Verification items for the finished model (mm, model axes). Coordinates: 2 decimals unless noted, no trailing zeros. Write each loop counter-clockwise with the first axis right and the second up, starting at its lowest first coordinate (ties: lowest second). Pieces come first, ordered by that corner, then holes. Notation, with made-up numbers: (-12.75, -21.75) -> (9.25, -21.75) arc R20 ccw to (9.25, 4.25) -> close; hole circle Ø6 at (79, 23). An arc over 180 degrees is marked (long way). Use CSV: the item, a comma, the result in double quotes.
Autodesk Inventor part; units mm, degrees
ref_plane "YZ Plane" through (0, 0, 0) normal (1, 0, 0) x (0, 1, 0)
ref_plane "XZ Plane" through (0, 0, 0) normal (0, 1, 0) x (-1, 0, 0)
ref_plane "XY Plane" through (0, 0, 0) normal (0, 0, 1) x (1, 0, 0)
sketch "Sketch1" plane through (0, 0, 0) normal (0, 0, 1) x (1, 0, 0)
  line L0 (51.9615, 90) -> (103.923, 0)
  line L1 (103.923, 0) -> (51.9615, -90)
  line L2 (51.9615, -90) -> (-51.9615, -90)
  line L3 (-51.9615, -90) -> (-103.923, 0)
  line L4 (-103.923, 0) -> (-51.9615, 90)
  line L5 (-51.9615, 90) -> (51.9615, 90)
  circle A0 centre (0, 0) radius 85
  circle A1 centre (0, 0) radius 10
  dimension "d1" = 170
  dimension "d2" = 180
  dimension "d12" = 20
extrude "Extrusion1" add sketch "Sketch1" along normal blind 1.6 contours L0 L1 L2 L3 L4 L5 | A0
sketch "Sketch3" plane through (0, 0, 1.6) normal (0, 0, 1) x (1, 0, 0)
  circle A0 centre (0, 0) radius 10
  circle A1 centre (-96, 0) radius 1.6
  line L0 (-51.9615, 90) -> (-103.923, 0)
  line L1 (-103.923, 0) -> (-51.9615, -90)
  arc A2 (-101.2676, 4.5994) -> (-101.2676, -4.5994) centre (-93.3013, 0) ccw
  dimension "d13" = 96
  dimension "d14" = 3.2
  dimension "d20" = 9.1987
  dimension "d21" = 93.3013
extrude "Extrusion3" cut sketch "Sketch3" against normal up to next contours A1 | A2 L1 L0
pattern_circular "Circular Pattern1" count 6 over 360 about axis through (0, 0, 0) along (0, 0, 1) of "Extrusion3"
sketch "Sketch4" plane through (0, 0, 1.6) normal (0, 0, 1) x (1, 0, 0)
  circle A0 centre (0, 0) radius 10
  circle A1 centre (0, 0) radius 85
  dimension "d22" = 170
extrude "Extrusion4" add sketch "Sketch4" along normal blind 0.1
properties part number "Heatbed_170mm_Hex"
1) Cross-section at C-C (x = -88). Record the boundary of the cut face in (y, z), plus the area to 3 significant figures.
Return value:
outline,"(-27.58, 0) -> (27.58, 0) -> (27.58, 1.6) -> (-27.58, 1.6) -> close"
area,"88.3 mm2"
2) Cross-section at D-D (y = -64). Record the boundary of the cut face in (x, z).
Return value:
outline,"(-66.97, 0) -> (66.97, 0) -> (66.97, 1.6) -> (55.94, 1.6) -> (55.94, 1.7) -> (-55.94, 1.7) -> (-55.94, 1.6) -> (-66.97, 1.6) -> close"
3) Gauge pin test, flat end, axial feed: pin 1 (4 mm diameter, centred on x = 48, y = 83.14, fed in from +Z). Record the tip position at first contact, or that the pin passes through.
Return value:
pin 1,"z = 1.6"
4) Mould release check, pull along Y, two halves, no side actions. Record for faces 1 (the flat face through (-1, -18, 1.7)), 2 (the cylindrical face through (51.308, 88.734, 0.811)), 3 (the cylindrical face through (-51.308, -88.734, 0.811)), 4 (the cylindrical face through (-2.17, 9.76, 0.84)): released by +Y, released by -Y, zero draft, split by the parting line, or undercut.
Return value:
face 1,"zero draft"
face 2,"released by +Y"
face 3,"released by -Y"
face 4,"undercut"
5) Cross-section at B-B (y = -44). Record the boundary of the cut face in (x, z).
Return value:
outline,"(-78.52, 0) -> (78.52, 0) -> (78.52, 1.6) -> (72.73, 1.6) -> (72.73, 1.7) -> (-72.73, 1.7) -> (-72.73, 1.6) -> (-78.52, 1.6) -> close"
6) Scan lines: L1, parallel to Z at x = 82.5, y = -27.5; L2, parallel to Y at x = 8, z = 1.4; L3, parallel to Y at x = 48, z = 0.5. Record each from-to range of solid material in increasing order.
Return value:
L1,"0 to 1.6"
L2,"-90 to -6, 6 to 90"
L3,"-89.9 to -84.74, -81.54 to 81.54, 84.74 to 89.9"
7) Cross-section at A-A (x = 0). Record the boundary of the cut face in (y, z).
Return value:
outline,"(-90, 0) -> (-10, 0) -> (-10, 1.7) -> (-85, 1.7) -> (-85, 1.6) -> (-90, 1.6) -> close; (10, 0) -> (90, 0) -> (90, 1.6) -> (85, 1.6) -> (85, 1.7) -> (10, 1.7) -> close"
